The listing builds one solid part. Answer for the finished solid, in the listing's coordinates (mm). Face numbers are marked on the shaded views. Round coordinates to 2 decimals unless told otherwise and drop trailing zeros. Write each loop counter-clockwise with the first axis right and the second up, starting at its lowest first coordinate (ties: lowest second). Pieces come first, ordered by that corner, then holes.
Autodesk Inventor part; units mm, degrees
ref_plane "YZ Plane" through (0, 0, 0) normal (1, 0, 0) x (0, 1, 0)
ref_plane "XZ Plane" through (0, 0, 0) normal (0, 1, 0) x (-1, 0, 0)
ref_plane "XY Plane" through (0, 0, 0) normal (0, 0, 1) x (1, 0, 0)
sketch "スケッチ1" plane through (0, 0, 0) normal (0, 1, 0) x (-1, 0, 0)
  line L0 (0, 0) -> (-62, 0)
  line L1 (-62, 0) -> (-62, 38)
  line L2 (-62, 38) -> (0, 38)
  line L3 (0, 38) -> (0, 0)
  line L4 (0, 19) -> (-8, 19)
  line L5 (-8, 19) -> (-8, 34)
  line L6 (-8, 34) -> (-18, 34)
  line L7 (-18, 34) -> (-28, 34)
  line L8 (-28, 34) -> (-38, 34)
  line L9 (-38, 34) -> (-48, 34)
  line L10 (-48, 34) -> (-58, 34)
  line L11 (-8, 4) -> (-18, 4)
  line L12 (-18, 4) -> (-28, 4)
  line L13 (-28, 4) -> (-38, 4)
  line L14 (-38, 4) -> (-48, 4)
  line L15 (-48, 4) -> (-58, 4)
  circle A0 centre (-58, 34) radius 1.5
  circle A1 centre (-48, 34) radius 1.5
  circle A2 centre (-38, 34) radius 1.5
  circle A3 centre (-28, 34) radius 1.5
  circle A4 centre (-18, 34) radius 1.5
  circle A5 centre (-8, 34) radius 1.5
  circle A6 centre (-58, 4) radius 1.5
  circle A7 centre (-48, 4) radius 1.5
  circle A8 centre (-38, 4) radius 1.5
  circle A9 centre (-28, 4) radius 1.5
  circle A10 centre (-18, 4) radius 1.5
  circle A11 centre (-8, 4) radius 1.5
  dimension "d0" = 62
  dimension "d1" = 38
  dimension "d2" = 8
  dimension "d3" = 15
  dimension "d4" = 10
  dimension "d5" = 10
  dimension "d6" = 10
  dimension "d7" = 10
  dimension "d8" = 10
  dimension "d9" = 3
  dimension "d10" = 3
  dimension "d11" = 3
  dimension "d12" = 3
  dimension "d13" = 3
  dimension "d14" = 3
extrude "押し出し1" add sketch "スケッチ1" along normal blind 7
properties part number "知能ロボコンギアボックススペーサ" material "ABS プラスチック"
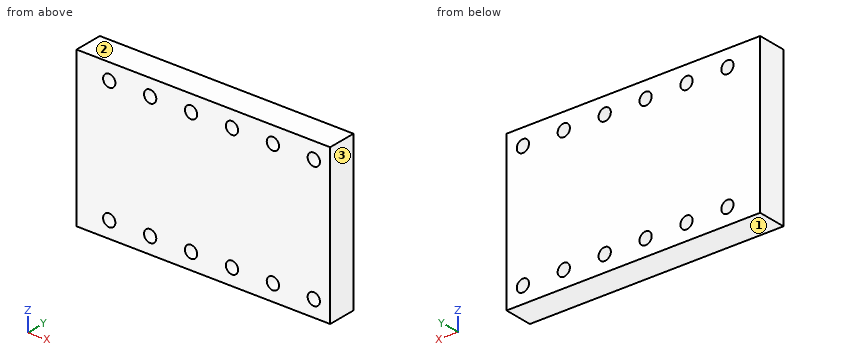
1. Section C-C on x = 27.5 is taken. Determine the outline of the cut face in (y, z), plus the area to 3 significant figures.
Geometry says:
outline: (0, 0) - (7, 0) - (7, 2.59) - (0, 2.59) - close; (0, 5.41) - (7, 5.41) - (7, 32.59) - (0, 32.59) - close; (0, 35.41) - (7, 35.41) - (7, 38) - (0, 38) - close
area: 226 mm2
2. A straight line is drawn through the part: line 1 along Z through (x, y) = (8, 4.25). Find the intervals that lie inside material, in ascending order.
Geometry says:
line 1: z = 0 to 2.5, 5.5 to 32.5, 35.5 to 38
3. Section A-A on x = 8 is taken. Determine the outline of the cut face in (y, z).
Geometry says:
outline: (0, 0) - (7, 0) - (7, 2.5) - (0, 2.5) - close; (0, 5.5) - (7, 5.5) - (7, 32.5) - (0, 32.5) - close; (0, 35.5) - (7, 35.5) - (7, 38) - (0, 38) - close
4. For a pull along Z with two mould halves and no side action, classify the marked faces 1, 2 and 3 as released by +Z, released by -Z, zero draft, split by the parting line, or undercut.
Geometry says:
face 1: released by -Z
face 2: released by +Z
face 3: zero draft
5. Section B-B on y = 5 is taken. Give the number of separate pieces and of enclosed holes in the cut face, plus the area to 3 significant figures.
Geometry says:
separate pieces: 1
enclosed holes: 12
area: 2,270 mm2
